Here's how the part is built. I have some questions about the finished solid (model axes, mm). Give positions to 0.01 mm unless a question says otherwise; leave off trailing zeros. Loops run counter-clockwise (first coordinate to the right, second up) from the corner with the lowest first, then second, coordinate; pieces in that order, holes last.
Q1. I need wall thicknesses on line 1 (X direction, y = 2, z = -20); line 2 (X direction, y = 0.9, z = -20); line 3 (Z direction, x = -17, y = 2.5). Which ranges of each line are inside material? Lowest first, please.
Q2. If we section it at B-B (z = -20): Give the number of separate pieces and of enclosed holes in the cut face, plus the area to 3 significant figures.
Q3. We'd pull the mould along Z, two halves only. Please class faces 1 (the face through (0, 0, -14)), 2 (the face through (-16.034, 1.972, -20.521)): +Z half, -Z half, draft (parallel to the pull), parting line (faces both ways), or undercut.
Q4. If we section it at C-C (y = 2.8): Please give me the cut outline in (x, z).
Q5. Will these pins go through, and if not, where does the flat tip stop? P1, Ø1, axis at x = -4.5, z = -18, coming from the -Y side; P2, Ø1, axis at y = 3, z = -20, coming from the +X side; P3, Ø1, axis at y = 3, z = -9.5, coming from the -X side; P4, Ø1.5, axis at y = 3, z = -15.5, coming from the +X side.
from build123d import *

# Parameters (mm, degrees)
SKETCH1_R           = 5
SKETCH1_R_2         = 4
BOSS_EXTRUDE1_DEPTH = 4
FILLET1_R           = 2


with BuildPart() as part:
    # Sketch1 → Boss-Extrude1 (new body)
    with BuildSketch(Plane(origin=(0, 0, 0), x_dir=(1, 0, 0), z_dir=(0, 1, 0))):
        with BuildLine():
            ThreePointArc((-20, 29), (-29, 20), (-20, 11))
            ThreePointArc((-20, 11), (-13.164114328, 7.468842596), (-9.989400339, 0.460305187))
            ThreePointArc((-9.989400339, 0.460305187), (0, -10), (9.989400339, 0.460305187))
            ThreePointArc((9.989400339, 0.460305187), (13.164114328, 7.468842596), (20, 11))
            ThreePointArc((20, 11), (29, 20), (20, 29))
            ThreePointArc((20, 29), (0, 26.863188813), (-20, 29))
        make_face()
        with Locations(Location((0, 0, 0), (0, 0, 270))):
            Circle(SKETCH1_R, mode=Mode.SUBTRACT)
        with Locations(Location((-20, 20, 0), (0, 0, 270))):
            Circle(SKETCH1_R_2, mode=Mode.SUBTRACT)
        with Locations(Location((20, 20, 0), (0, 0, 270))):
            Circle(SKETCH1_R_2, mode=Mode.SUBTRACT)
    extrude(amount=BOSS_EXTRUDE1_DEPTH)

    # Fillet1
    fillet1_edges = [part.edges().sort_by_distance(p)[0] for p in [
        (13.164114328, 4, -7.468842596),
        (-20, 2, -11),
        (-20, 2, -29),
        (20, 2, -29),
        (20, 2, -11),
        (9.989400339, 2, -0.460305187),
        (-9.989400339, 2, -0.460305187),
        (29, 4, -20),
        (0, 4, -26.863188813),
        (-29, 4, -20),
        (-13.164114328, 4, -7.468842596),
        (-29, 0, -20),
        (0, 0, -26.863188813),
        (29, 0, -20),
        (0, 4, 10),
        (13.164114328, 0, -7.468842596),
        (0, 0, 10),
        (-13.164114328, 0, -7.468842596),
    ]]
    fillet(fillet1_edges, radius=FILLET1_R - 0.0001)  # a hair under: the kernel refuses the full size


solid = part.part
Check sheet entries:
1. line 1: x = -29 to -24, -16 to 16, 24 to 29
1. line 2: x = -28.67 to -24, -16 to 16, 24 to 28.67
1. line 3: z = -28.34 to -22.65, -17.35 to -10.22
2. separate pieces: 3
2. enclosed holes: 0
2. area: 165 mm2
3. face 1: draft
3. face 2: undercut
4. outline: (-20.25, -28.83) arc R1.83 ccw to (-19.82, -28.79) arc R94.83 cw to (19.82, -28.79) arc R1.83 ccw to (20.25, -28.83) arc R8.83 ccw to (20.13, -11.17) arc R2.17 cw to (19.82, -11.14) arc R11.89 cw to (9.84, -0.63) arc R2.17 cw to (9.83, -0.33) arc R9.83 ccw (long way) to (-9.83, -0.33) arc R2.17 cw to (-9.84, -0.63) arc R11.89 cw to (-19.82, -11.14) arc R2.17 cw to (-20.13, -11.17) arc R8.83 ccw to start; hole circle Ø8 at (-20, -20); hole circle Ø10 at (0, 0); hole circle Ø8 at (20, -20)
5. P1: stops at y = 0
5. P2: stops at x = 28.94
5. P3: stops at x = -16.21
5. P4: stops at x = 28.03
